Part model, mm, in its own coordinate system. A direction names the side the tool comes from. Round coordinates to 2 decimals unless told otherwise and drop trailing zeros. Loops run counter-clockwise (first coordinate to the right, second up) from the corner with the lowest first, then second, coordinate; pieces in that order, holes last.
(1) Cut at B-B on z = 0.7. Count the separate pieces of the cut face and the enclosed holes in it, then the cut area to 3 significant figures.
(2) Probe probe 1 along X at (y, z) = (69, 2.05); probe 2 along X at (y, z) = (37, 1.85); probe 3 along Y at (x, z) = (-150, 0.35). List the from-to ranges inside material, lowest first.
(3) Mould opens along Y. For faces 1 (the face through (-176.299, 75.598, 1.521)), 2 (the face through (-138.763, 42.049, 1.479)), 3 (the face through (-65, 11, 1)) say: +Y half, -Y half, draft (parallel to the pull), parting line (faces both ways), or undercut.
(4) Cut at A-A on y = 57. List the corners of the cut face in (x, z).
(5) Flat gauge pins, fed straight in: pin 1 (4 mm diameter, centred on x = -154.01, y = 57, fed in from +Z); pin 2 (0.9 mm diameter, centred on x = -153.5, z = 2, fed in from -Y); pin 3 (1.5 mm diameter, centred on x = -122, z = 1.5, fed in from -Y); pin 4 (1.5 mm diameter, centred on x = -79, z = 1, fed in from +Y). Where does each tip first touch, or does it go through?
(6) Tool access for faces 4 (the face through (-76, 3, 1)), 5 (the face through (-115.155, 68, 2)): list every direction of +Z, -Z, +X, -X, +Y, -Y with a clear straight run to the whole face (end or side of a thin tool).
from build123d import *

# Parameters (mm, degrees)
EXTRUDE_1_DEPTH     = 3
SKETCH_3_R          = 1.6
CUT_EXTRUDE_1_DEPTH = 10
SKETCH_4_R          = 1.6
CUT_EXTRUDE_2_DEPTH = 10
SKETCH_5_R          = 2
CUT_EXTRUDE_3_DEPTH = 10
SKETCH_6_R          = 1.6
CUT_EXTRUDE_4_DEPTH = 3
SKETCH_7_R          = 1.6
CUT_EXTRUDE_5_DEPTH = 3
FILLET_1_R          = 2
CUT_EXTRUDE_6_DEPTH = 11.6
FILLET_2_R          = 3
CUT_EXTRUDE_7_DEPTH = 11.6
EXTRUDE_2_DEPTH     = 3
CUT_EXTRUDE_8_DEPTH = 193.98963408
FILLET_3_R          = 2
FILLET_4_R          = 2


with BuildPart() as part:
    # 草图2 → 凸台-拉伸1 (new body)
    with BuildSketch(Plane.XY):
        with BuildLine():
            Line((-177.154590294, 76.5), (-177.154590294, 66.5))
            ThreePointArc((-177.154590294, 66.5), (-154.308919227, 11.345671067), (-99.154590294, -11.5))
            Line((-99.154590294, -11.5), (-88, -11.5))
            Line((-88, -11.5), (-65, -11.5))
            Line((-65, -11.5), (-65, -3))
            Line((-65, -3), (-88, -3))
            Line((-88, -3), (-88, 3))
            Line((-88, 3), (-65, 3))
            Line((-65, 3), (-65, 17.056624327))
            Line((-65, 17.056624327), (-62.5, 18.5))
            Line((-62.5, 18.5), (-62.5, 34.5))
            Line((-62.5, 34.5), (-65, 35.943375673))
            Line((-65, 35.943375673), (-65, 50))
            Line((-65, 50), (-107.154590294, 50))
            Line((-107.154590294, 50), (-107.154590294, 76.5))
            Line((-107.154590294, 76.5), (-177.154590294, 76.5))
        make_face()
    extrude(amount=EXTRUDE_1_DEPTH)

    # 草图3 → 切除-拉伸1 (cut)
    with BuildSketch(Plane.XY.offset(3)):
        with Locations((-142, 6)):
            Circle(SKETCH_3_R)
        with Locations((-122, 6)):
            Circle(SKETCH_3_R)
    extrude(amount=-CUT_EXTRUDE_1_DEPTH, mode=Mode.SUBTRACT)

    # 草图4 → 切除-拉伸2 (cut)
    with BuildSketch(Plane.XY.offset(3)):
        with Locations((-170.287955794, 46.10283567)):
            Circle(SKETCH_4_R)
        with Locations((-159.021847878, 23.00389133)):
            Circle(SKETCH_4_R)
        with Locations((-114.540055415, -5.882922454)):
            Circle(SKETCH_4_R)
        with Locations((-93.154590294, -7.5)):
            Circle(SKETCH_4_R)
    extrude(amount=-CUT_EXTRUDE_2_DEPTH, mode=Mode.SUBTRACT)

    # 草图5 → 切除-拉伸3 (cut)
    with BuildSketch(Plane.XY.offset(3)):
        with Locations((-86, 3)):
            Circle(SKETCH_5_R)
        with Locations((-86, -3)):
            Circle(SKETCH_5_R)
    extrude(amount=-CUT_EXTRUDE_3_DEPTH, mode=Mode.SUBTRACT)

    # 草图6 → 切除-拉伸4 (cut)
    with BuildSketch(Plane.XY.offset(3)):
        with Locations((-111.154590294, 72.5)):
            Circle(SKETCH_6_R)
        with Locations((-111.154590294, 64.5)):
            Circle(SKETCH_6_R)
    extrude(amount=-CUT_EXTRUDE_4_DEPTH, mode=Mode.SUBTRACT)

    # 草图7 → 切除-拉伸5 (cut)
    with BuildSketch(Plane.XY.offset(3)):
        with Locations((-154.010091835, 57)):
            Circle(SKETCH_7_R)
        with Locations((-122.010091835, 57)):
            Circle(SKETCH_7_R)
    extrude(amount=-CUT_EXTRUDE_5_DEPTH, mode=Mode.SUBTRACT)

    # 圆角1
    fillet_1_edges = [part.edges().sort_by_distance(p)[0] for p in [
        (-107.154590294, 50, 1.5),
    ]]
    fillet(fillet_1_edges, radius=FILLET_1_R)

    # 草图8 → 切除-拉伸6 (cut)
    with BuildSketch(Plane.XY.offset(3)):
        Polygon((-95, 50), (-87, 42), (-65, 42), (-65, 50), align=None)
    extrude(amount=-CUT_EXTRUDE_6_DEPTH, mode=Mode.SUBTRACT)

    # 圆角2
    fillet_2_edges = [part.edges().sort_by_distance(p)[0] for p in [
        (-95, 50, 1.5),
        (-65, 42, 1.5),
        (-87, 42, 1.5),
        (-177.154590294, 76.5, 1.5),
        (-65, -11.5, 1.5),
        (-65, -3, 1.5),
        (-65, 3, 1.5),
        (-107.154590294, 76.5, 1.5),
    ]]
    fillet(fillet_2_edges, radius=FILLET_2_R)

    # 草图9 → 切除-拉伸7 (cut)
    with BuildSketch(Plane.XY.offset(3)):
        with BuildLine():
            ThreePointArc((-145.154590294, 66.5), (-145.072019197, 63.745054808), (-144.824602337, 61))
            Line((-144.824602337, 61), (-172.154590294, 61))
            Line((-172.154590294, 61), (-172.154590294, 72.5))
            Line((-172.154590294, 72.5), (-145.154590294, 72.5))
            Line((-145.154590294, 72.5), (-145.154590294, 66.5))
        make_face()
        with BuildLine():
            Line((-133.154590294, 72.5), (-133.154590294, 66.5))
            ThreePointArc((-133.154590294, 66.5), (-133.042454912, 63.740900214), (-132.706788434, 61))
            Line((-132.706788434, 61), (-121.498246805, 61))
            Line((-121.498246805, 61), (-115.154590294, 65.382793706))
            Line((-115.154590294, 65.382793706), (-115.154590294, 72.5))
            Line((-115.154590294, 72.5), (-133.154590294, 72.5))
        make_face()
        with BuildLine():
            Line((-127.680893946, 48), (-111.060471194, 48))
            ThreePointArc((-111.060471194, 48), (-105.946714568, 45.574727054), (-100.383436414, 44.53434642))
            Line((-100.383436414, 44.53434642), (-99.407755019, 32.500942548))
            ThreePointArc((-99.407755019, 32.500942548), (-115.498385615, 36.685903426), (-127.680893946, 48))
        make_face()
        with BuildLine():
            Line((-166.665700491, 48), (-141.270501777, 48))
            ThreePointArc((-141.270501777, 48), (-139.774924791, 44.913234948), (-138.053500491, 41.946491381))
            Line((-138.053500491, 41.946491381), (-157.497103519, 27.819886884))
            ThreePointArc((-157.497103519, 27.819886884), (-162.885217731, 37.544739224), (-166.665700491, 48))
        make_face()
        with BuildLine():
            ThreePointArc((-123.234931322, 27.306414096), (-117.609516434, 24.364317958), (-111.632610014, 22.224735756))
            Line((-111.632610014, 22.224735756), (-114.443614375, 9))
            Line((-114.443614375, 9), (-136.199324912, 9))
            Line((-136.199324912, 9), (-123.234931322, 27.306414096))
        make_face()
        with BuildLine():
            ThreePointArc((-105.763724409, 20.977265611), (-102.467762347, 20.619471549), (-99.154590294, 20.5))
            Line((-99.154590294, 20.5), (-98.434705623, 20.5))
            Line((-98.434705623, 20.5), (-96.488759677, -3.5))
            Line((-96.488759677, -3.5), (-99.154590294, -3.5))
            ThreePointArc((-99.154590294, -3.5), (-104.977776216, -3.257368827), (-110.760593955, -2.531157306))
            Line((-110.760593955, -2.531157306), (-105.763724409, 20.977265611))
        make_face()
        with BuildLine():
            ThreePointArc((-134.526788978, 37.092389415), (-131.483826087, 33.776606028), (-128.131412478, 30.774046183))
            Line((-128.131412478, 30.774046183), (-142.021368274, 11.160688967))
            ThreePointArc((-142.021368274, 11.160688967), (-148.351253457, 16.703530912), (-153.970392005, 22.965784918))
            Line((-153.970392005, 22.965784918), (-134.526788978, 37.092389415))
        make_face()
        Polygon((-69.56341496, 38), (-66.387988479, 32.5), (-93.387988479, 32.5), (-93.833934425, 38), align=None)
        Polygon((-91.320420912, 7), (-69, 7), (-69, 20.5), (-92.415015506, 20.5), align=None)
    extrude(amount=-CUT_EXTRUDE_7_DEPTH, mode=Mode.SUBTRACT)

    # 草图13 → 凸台-拉伸2 (add)
    with BuildSketch(Plane.XY.offset(3)):
        with BuildLine():
            Line((-74.049844719, 34.211145618), (-77.472135955, 32.5))
            Line((-77.472135955, 32.5), (-73, 32.5))
            Line((-73, 32.5), (-67.86914014, 35.06542993))
            Line((-67.86914014, 35.06542993), (-68.870939906, 36.800598024))
            Line((-68.870939906, 36.800598024), (-69.56341496, 38))
            Line((-69.56341496, 38), (-74.94427191, 38))
            ThreePointArc((-74.94427191, 38), (-72.997773931, 36.459505841), (-74.049844719, 34.211145618))
        make_face()
        Polygon((-79.708203932, 20.5), (-73, 20.5), (-69, 18.5), (-69, 15.145898034), align=None)
    extrude(amount=-EXTRUDE_2_DEPTH)

    # 草图11 → 切除-拉伸8 (cut, through all)
    with BuildSketch(Plane.XY.offset(3)):
        Polygon((-65, 36.5), (-85, 26.5), (-65, 16.5), (-59.800529593, 16.5), (-59.800529593, 36.5), align=None)
    extrude(amount=-CUT_EXTRUDE_8_DEPTH, mode=Mode.SUBTRACT)

    # 圆角3
    fillet_3_edges = [part.edges().sort_by_distance(p)[0] for p in [
        (-111.632610014, 22.224735756, 1.5),
        (-114.443614375, 9, 1.5),
        (-136.199324912, 9, 1.5),
        (-123.234931322, 27.306414096, 1.5),
        (-111.060471194, 48, 1.5),
        (-100.383436414, 44.53434642, 1.5),
        (-99.407755019, 32.500942548, 1.5),
        (-127.680893946, 48, 1.5),
        (-115.154590294, 72.5, 1.5),
        (-115.154590294, 65.382793706, 1.5),
        (-121.498246805, 61, 1.5),
        (-132.706788434, 61, 1.5),
        (-133.154590294, 72.5, 1.5),
        (-128.131412478, 30.774046183, 1.5),
        (-142.021368274, 11.160688967, 1.5),
        (-153.970392005, 22.965784918, 1.5),
        (-134.526788978, 37.092389415, 1.5),
        (-144.824602337, 61, 1.5),
        (-172.154590294, 61, 1.5),
        (-172.154590294, 72.5, 1.5),
        (-145.154590294, 72.5, 1.5),
        (-92.415015506, 20.5, 1.5),
        (-69, 15.145898034, 1.5),
        (-69, 7, 1.5),
        (-91.320420912, 7, 1.5),
        (-98.434705623, 20.5, 1.5),
        (-96.488759677, -3.5, 1.5),
        (-110.760593955, -2.531157306, 1.5),
        (-105.763724409, 20.977265611, 1.5),
        (-141.270501777, 48, 1.5),
        (-138.053500491, 41.946491381, 1.5),
        (-157.497103519, 27.819886884, 1.5),
        (-166.665700491, 48, 1.5),
        (-93.387988479, 32.5, 1.5),
        (-93.833934425, 38, 1.5),
        (-77.472135955, 32.5, 1.5),
        (-79.708203932, 20.5, 1.5),
    ]]
    fillet(fillet_3_edges, radius=FILLET_3_R)

    # 圆角4
    fillet_4_edges = [part.edges().sort_by_distance(p)[0] for p in [
        (-65, 16.5, 1.5),
        (-85, 26.5, 1.5),
        (-65, 36.5, 1.5),
    ]]
    fillet(fillet_4_edges, radius=FILLET_4_R)


solid = part.part
Final values:
1. separate pieces: 1
1. enclosed holes: 19
1. area: 4,470 mm2
2. probe 1: x = -177.15 to -172.15, -145.15 to -133.15, -115.15 to -107.15
2. probe 2: x = -171.36 to -162.63, -144.86 to -116.06, -99.77 to -93.4, -73.21 to -65.14
2. probe 3: y = 7.35 to 18.39, 25.85 to 33.27, 48 to 61, 72.5 to 76.5
3. face 1: +Y half
3. face 2: undercut
3. face 3: draft
4. outline: (-176.57, 0) - (-155.61, 0) - (-155.61, 3) - (-176.57, 3) - close; (-152.41, 0) - (-123.61, 0) - (-123.61, 3) - (-152.41, 3) - close; (-120.41, 0) - (-107.15, 0) - (-107.15, 3) - (-120.41, 3) - close
5. pin 1: stops at z = 3
5. pin 2: stops at y = 10.11
5. pin 3: stops at y = -8.31
5. pin 4: stops at y = 42
6. face 4: +Z, -Z, +X
6. face 5: +Z, -Z
